```python
from build123d import *

# Parameters (mm, degrees)
SKETCH2_R           = 2
BOSS_EXTRUDE1_DEPTH = 5
CUT_EXTRUDE1_DEPTH  = 2


with BuildPart() as part:
    # Sketch2 → Boss-Extrude1 (new body)
    # profile 1 of 2: a face of its own
    with BuildSketch(Plane(origin=(0, 0, 0), x_dir=(1, 0, 0), z_dir=(0, 1, 0))):
        with BuildLine():
            ThreePointArc((37.5, -45.5), (36.085786438, -42.085786438), (39.5, -43.5))
            Line((39.5, -43.5), (47.5, -43.5))
            Line((47.5, -43.5), (47.5, 53.5))
            Line((47.5, 53.5), (-47.5, 53.5))
            Line((-47.5, 53.5), (-47.5, -53.5))
            Line((-47.5, -53.5), (37.5, -53.5))
            Line((37.5, -53.5), (37.5, -45.5))
        make_face()
        with Locations(Location((-37.5, -43.5, 0), (0, 0, 270))):
            Circle(SKETCH2_R, mode=Mode.SUBTRACT)
        with Locations(Location((-37.5, 43.5, 0), (0, 0, 270))):
            Circle(SKETCH2_R, mode=Mode.SUBTRACT)
        with Locations(Location((37.5, 43.5, 0), (0, 0, 270))):
            Circle(SKETCH2_R, mode=Mode.SUBTRACT)
    # profile 2 of 2: a face of its own
    with BuildSketch(Plane(origin=(0, 0, 0), x_dir=(1, 0, 0), z_dir=(0, 1, 0))):
        with BuildLine():
            Line((47.5, -43.5), (39.5, -43.5))
            ThreePointArc((39.5, -43.5), (38.914213562, -44.914213562), (37.5, -45.5))
            Line((37.5, -45.5), (37.5, -53.5))
            Line((37.5, -53.5), (47.5, -53.5))
            Line((47.5, -53.5), (47.5, -43.5))
        make_face()
    extrude(amount=BOSS_EXTRUDE1_DEPTH)

    # Sketch3 → Cut-Extrude1 (cut)
    with BuildSketch(Plane(origin=(0, 5, 0), x_dir=(1, 0, 0), z_dir=(0, 1, 0))):
        Polygon((-47.5, 40.237063088), (-47.5, 17.240159463), (-47.5, 17.140159463), (-30.489963443, 17.140159463), (-30.489963443, 37.232769094), (-32.282228416, 40.337063088), (-47.5, 40.337063088), align=None)
        Polygon((47.5, 40.337063088), (32.282228416, 40.337063088), (30.489963443, 37.232769094), (30.489963443, 17.140159463), (47.5, 17.140159463), (47.5, 17.240159463), (47.5, 40.237063088), align=None)
        Polygon((47.5, -17.240159463), (47.5, -17.140159463), (30.489963443, -17.140159463), (30.489963443, -37.232769094), (32.282228416, -40.337063088), (47.5, -40.337063088), (47.5, -40.237063088), align=None)
        Polygon((-30.489963443, -17.140159463), (-47.5, -17.140159463), (-47.5, -17.240159463), (-47.5, -40.237063088), (-47.5, -40.337063088), (-32.282228416, -40.337063088), (-30.489963443, -37.232769094), align=None)
    extrude(amount=-CUT_EXTRUDE1_DEPTH, mode=Mode.SUBTRACT)


solid = part.part
```
Source: CAD feature listing. Evaluate the final solid. Frame: model axes, mm. A direction names the side the tool comes from. Give positions to 0.01 mm unless a question says otherwise; leave off trailing zeros. Loops run counter-clockwise (first coordinate to the right, second up) from the corner with the lowest first, then second, coordinate; pieces in that order, holes last. Notation, with made-up numbers: (-2.75, -30.75) -> (39.25, -30.75) arc R19 cw to (39.25, -0.75) -> close; hole circle Ø1 at (-40, 45.25). An arc over 180 degrees is marked (long way). Put each result on its own line as item: value. Start each with the question number.
1) Contact query for flat-ended pins moving along their axis: P1, Ø0.6, axis at y = 4, z = -27, coming from the +X side; P2, Ø1, axis at y = 4, z = -30.5, coming from the -X side; P3, Ø1.5, axis at x = 33.5, z = -22, coming from the -Y side; P4, Ø8.5, axis at x = 42, z = -29.5, coming from the +Y side. Output: stop coordinate, or through.
2) Cut plane C-C (z = 23). Return loops of the section in (x, y).
3) Material intervals for probe 1 along X at (y, z) = (3.6, 43.5); probe 2 along X at (y, z) = (1.3, -45); probe 3 along X at (y, z) = (4.5, -26), sorted ascending.
4) Cut plane A-A (x = -37.5). Return loops of the section in (y, z).
5) Reachability of faces 1 (the face through (-39.452, 2.465, 43.066)), 2 (the face through (39, 3, 29)), 3 (the face through (-39, 3, -29)) from +Z, -Z, +X, -X, +Y, -Y: full face, straight path, thin tool, end or side. Return the list, or none.
6) Draft query along X for faces 4 (the face through (47.5, 2, 1)), 5 (the face through (35.548, 2.465, -43.934)), 6 (the face through (-1, 0, -1)). Return one class per face: released by +X, released by -X, zero draft, split by the parting line, or undercut.
7) Cut plane B-B (z = -43.5). Return loops of the section in (x, y).
Results are:
1. P1: stops at x = 30.49
1. P2: stops at x = -30.49
1. P3: stops at y = 0
1. P4: stops at y = 3
2. outline: (-47.5, 0) -> (47.5, 0) -> (47.5, 3) -> (30.49, 3) -> (30.49, 5) -> (-30.49, 5) -> (-30.49, 3) -> (-47.5, 3) -> close
3. probe 1: x = -47.5 to -39.5, -35.5 to 35.5, 39.5 to 47.5
3. probe 2: x = -47.5 to -38.82, -36.18 to 36.18, 38.82 to 47.5
3. probe 3: x = -30.49 to 30.49
4. outline: (0, -53.5) -> (5, -53.5) -> (5, -45.5) -> (0, -45.5) -> close; (0, -41.5) -> (5, -41.5) -> (5, -40.34) -> (3, -40.34) -> (3, -17.14) -> (5, -17.14) -> (5, 17.14) -> (3, 17.14) -> (3, 40.34) -> (5, 40.34) -> (5, 41.5) -> (0, 41.5) -> close; (0, 45.5) -> (5, 45.5) -> (5, 53.5) -> (0, 53.5) -> close
5. face 1: +Y, -Y
5. face 2: +X, +Y
5. face 3: -X, +Y
6. face 4: released by +X
6. face 5: undercut
6. face 6: zero draft
7. outline: (-47.5, 0) -> (-39.5, 0) -> (-39.5, 5) -> (-47.5, 5) -> close; (-35.5, 0) -> (35.5, 0) -> (35.5, 5) -> (-35.5, 5) -> close; (39.5, 0) -> (47.5, 0) -> (47.5, 5) -> (39.5, 5) -> close
